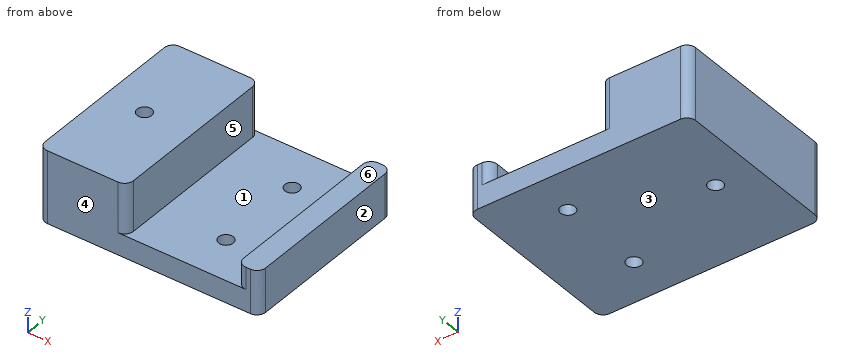
Autodesk Inventor part; units mm, degrees
ref_plane "YZ Plane" through (0, 0, 0) normal (1, 0, 0) x (0, 1, 0)
ref_plane "XZ Plane" through (0, 0, 0) normal (0, 1, 0) x (-1, 0, 0)
ref_plane "XY Plane" through (0, 0, 0) normal (0, 0, 1) x (1, 0, 0)
sketch "スケッチ1" plane through (0, 0, 0) normal (0, 0, 1) x (1, 0, 0)
  line L0 (22.5, -20) -> (-22.5, -20)
  line L1 (-22.5, -20) -> (-22.5, 20)
  line L2 (-22.5, 20) -> (22.5, 20)
  line L3 (22.5, 20) -> (22.5, -20)
  line L4 (22.5, -20) -> (-22.5, 20) construction
  line L5 (-22.5, -20) -> (22.5, 20) construction
  circle A0 centre (12.5, 10) radius 1.65
  circle A1 centre (12.5, -10) radius 1.65
  circle A2 centre (-13.5, 0) radius 1.65
  point P0 (0, 0)
  dimension "d0" = 45
  dimension "d1" = 40
  dimension "d2" = 3.3
  dimension "d3" = 3.3
  dimension "d4" = 10
  dimension "d5" = 10
  dimension "d6" = 10
  dimension "d7" = 10
  dimension "d8" = 3.3
  dimension "d9" = 36
  dimension "d10" = 20
extrude "押し出し1" add sketch "スケッチ1" along normal blind 5
sketch "スケッチ2" plane through (0, 0, 5) normal (0, 0, 1) x (1, 0, 0)
  line L0 (22.5, 20) -> (-22.5, 20)
  line L1 (-22.5, 20) -> (-22.5, -20)
  line L2 (-22.5, -20) -> (22.5, -20)
  line L3 (22.5, -20) -> (22.5, 20)
  circle A0 centre (-13.5, 0) radius 1.65
  circle A1 centre (12.5, -10) radius 1.65
  circle A2 centre (12.5, 10) radius 1.65
  line L4 (-22.5, 20) -> (0, 20)
  line L5 (0, 20) -> (0, -20)
  line L6 (0, -20) -> (-22.5, -20)
  line L7 (-22.5, -20) -> (-22.5, 20)
  line L8 (22.5, 20) -> (-22.5, 20)
  line L9 (-2.5, 20) -> (-2.5, -20)
  point P0 (0, 0)
  point P1 (-2.5, -20)
  dimension "d15" = 20
extrude "押し出し2" add sketch "スケッチ2" along normal blind 11.4 contours L9 L2 L1 L0
fillet "フィレット1" radius 2 4 edges at (-22.5, 20, 8.2) (-22.5, -20, 8.2) (-2.5, -20, 10.7) (-2.5, 20, 10.7)
sketch "スケッチ3" plane through (22.5, -20, 0) normal (1, 0, 0) x (0, 0, -1)
  line L0 (0, 0) -> (0, 40)
  line L1 (0, 40) -> (-5, 40)
  line L2 (-5, 0) -> (-5, 40)
  line L3 (0, 0) -> (-5, 0)
  line L4 (-5, 40) -> (-16.4, 40)
  line L5 (0, 0) -> (-10, 0)
  line L6 (-10, 0) -> (-10, 40)
  line L7 (-10, 40) -> (0, 40)
  line L8 (0, 40) -> (0, 0)
  point P0 (0, 20)
  dimension "d17" = 10
extrude "押し出し3" add sketch "スケッチ3" along normal blind 5
fillet "フィレット2" radius 2 4 edges at (27.5, 20, 5) (27.5, -20, 5) (22.5, 20, 7.5) (22.5, -20, 7.5)
properties part number "soroban_hold"
For this review, take the finished solid that the model builds, in its own axes (mm). Face numbers are marked on the shaded views. A direction names the side the tool comes from. Give positions to 0.01 mm unless a question says otherwise; leave off trailing zeros. Order: outer loops, then holes, each group sorted by start corner. A loop starts at its lowest first (then second) coordinate and runs counter-clockwise, first axis right, second up.
1) Take a section at B-B (x = -13.5). Give the boundary of the cut face in (y, z), then the cut area to 3 significant figures.
2) Take a section at C-C (z = 15.25). Give the boundary of the cut face in (x, y), then the cut area to 3 significant figures.
3) Insertion check: pin 1 (14.5 mm diameter, centred on x = 12.5, y = 5, fed in from +Z); pin 2 (2.5 mm diameter, centred on x = 25.5, y = -3.5, fed in from +Z). Each pin has a flat end and moves straight along its axis. Give the tip position at first contact, or say it passes through.
4) The part is to be moulded in two halves that separate along X. For the marked faces 1, 2 and 3, say which applies: released by +X, released by -X, zero draft, split by the parting line, or undercut.
5) For the marked faces 4, 5 and 6, list the 3-axis set-ups (+Z, -Z, +X, -X, +Y, -Y) from which the entire face can be reached by the end or side of a thin tool; tool diameter is ignored.
6) Take a section at A-A (z = 7.5). Give the boundary of the cut face in (x, y), then the cut area to 3 significant figures.
7) Take a section at D-D (y = 10). Give the boundary of the cut face in (x, z).
8) Wall thickness on line 1 (Y direction, x = 12.5, z = 3.25); line 2 (X direction, y = 16, z = 8.75); line 3 (Y direction, x = -13.5, z = 4): over which ranges is each line inside the solid? List them lowest first.
Derived:
1. outline: (-20, 0) - (-1.65, 0) - (-1.65, 16.4) - (-20, 16.4) - close; (1.65, 0) - (20, 0) - (20, 16.4) - (1.65, 16.4) - close
1. area: 602 mm2
2. outline: (-22.5, -18) arc R2 ccw to (-20.5, -20) - (-4.5, -20) arc R2 ccw to (-2.5, -18) - (-2.5, 18) arc R2 ccw to (-4.5, 20) - (-20.5, 20) arc R2 ccw to (-22.5, 18) - close; hole circle Ø3.3 at (-13.5, 0)
2. area: 788 mm2
3. pin 1: stops at z = 5
3. pin 2: stops at z = 10
4. face 1: undercut
4. face 2: released by +X
4. face 3: zero draft
5. face 4: +Z, -Z, +X, -X, -Y
5. face 5: +Z, +Y, -Y
5. face 6: +Z, +X, +Y, -Y
6. outline: (-22.5, -18) arc R2 ccw to (-20.5, -20) - (-4.5, -20) arc R2 ccw to (-2.5, -18) - (-2.5, 18) arc R2 ccw to (-4.5, 20) - (-20.5, 20) arc R2 ccw to (-22.5, 18) - close; (22.5, -18) arc R2 ccw to (24.5, -20) - (25.5, -20) arc R2 ccw to (27.5, -18) - (27.5, 18) arc R2 ccw to (25.5, 20) - (24.5, 20) arc R2 ccw to (22.5, 18) - close; hole circle Ø3.3 at (-13.5, 0)
6. area: 985 mm2
7. outline: (-22.5, 0) - (10.85, 0) - (10.85, 5) - (-2.5, 5) - (-2.5, 16.4) - (-22.5, 16.4) - close; (14.15, 0) - (27.5, 0) - (27.5, 10) - (22.5, 10) - (22.5, 5) - (14.15, 5) - close
8. line 1: y = -20 to -11.65, -8.35 to 8.35, 11.65 to 20
8. line 2: x = -22.5 to -2.5, 22.5 to 27.5
8. line 3: y = -20 to -1.65, 1.65 to 20
